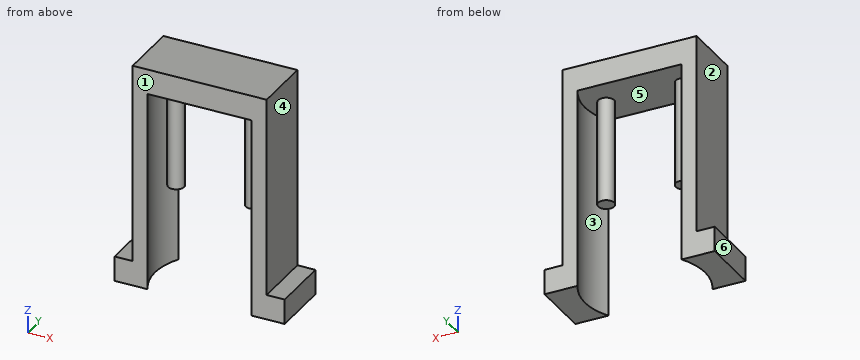
from build123d import *

# Parameters (mm, degrees)
BOSS_EXTRU_2_DEPTH = 5
BOSS_EXTRU_3_DEPTH = 35
ESQUISSE7_W        = 13.392304845
ESQUISSE7_H        = 12
ESQUISSE7_R        = 1.6
BOSS_EXTRU_4_DEPTH = 5
BOSS_EXTRU_5_START = -26
ESQUISSE9_R        = 1.6
BOSS_EXTRU_5_DEPTH = 26


with BuildPart() as part:
    # Esquisse5 → Boss.-Extru.2 (new body)
    with BuildSketch(Plane.XY):
        with BuildLine():
            Line((-17, 6), (-17, -6))
            Line((-17, -6), (-10.392304845, -6))
            ThreePointArc((-10.392304845, -6), (-12, 0), (-10.392304845, 6))
            Line((-10.392304845, 6), (-17, 6))
        make_face()
    boss_extru_2 = extrude(amount=BOSS_EXTRU_2_DEPTH)

    # Esquisse6 → Boss.-Extru.3 (add)
    with BuildSketch(Plane.XY.offset(5)):
        with BuildLine():
            Line((-13.392304845, 6), (-13.392304845, -6))
            Line((-13.392304845, -6), (-10.392304845, -6))
            ThreePointArc((-10.392304845, -6), (-12, 0), (-10.392304845, 6))
            Line((-10.392304845, 6), (-13.392304845, 6))
        make_face()
    boss_extru_3 = extrude(amount=BOSS_EXTRU_3_DEPTH)

    # Esquisse7 → Boss.-Extru.4 (add)
    with BuildSketch(Plane.XY.offset(40)):
        with Locations((-6.696152422, 0)):
            Rectangle(ESQUISSE7_W, ESQUISSE7_H)
        with Locations((-7.75, 0)):
            Circle(ESQUISSE7_R, mode=Mode.SUBTRACT)
    boss_extru_4 = extrude(amount=BOSS_EXTRU_4_DEPTH)

    # Symétrie9: Boss.-Extru.4 across plane
    add(boss_extru_4.mirror(Plane(origin=(0, 0, 0), x_dir=(0, 0, 1), z_dir=(1, 0, 0))))

    # Symétrie10: Boss.-Extru.3 across plane
    add(boss_extru_3.mirror(Plane(origin=(0, 0, 0), x_dir=(0, 0, 1), z_dir=(1, 0, 0))))

    # Symétrie11: Boss.-Extru.2 across plane
    add(boss_extru_2.mirror(Plane(origin=(0, 0, 0), x_dir=(0, 0, 1), z_dir=(1, 0, 0))))

    # Esquisse9 → Boss.-Extru.5 (add)
    with BuildSketch(Plane.XY.offset(45).offset(BOSS_EXTRU_5_START)):
        with Locations((-7.75, 0)):
            Circle(ESQUISSE9_R)
    boss_extru_5 = extrude(amount=BOSS_EXTRU_5_DEPTH)

    # Symétrie12: Boss.-Extru.5 across plane
    add(boss_extru_5.mirror(Plane(origin=(0, 0, 0), x_dir=(0, 0, 1), z_dir=(1, 0, 0))))


solid = part.part
Source: CAD feature listing. Evaluate the final solid. Frame: model axes, mm. Face numbers are marked on the shaded views. A direction names the side the tool comes from. Coordinates: 2 decimals unless noted, no trailing zeros. Order: outer loops, then holes, each group sorted by start corner. A loop starts at its lowest first (then second) coordinate and runs counter-clockwise, first axis right, second up. Notation, with made-up numbers: M 70.25,78.25 L 104.25,78.25 A12 cw 104.25,96.25 Z; hole C 30.25,-18 d5. An arc over 180 degrees is marked long. Write each question's results on one line, items separated by ' | '. Start each with the question number.
1. Section A-A, the plane z = 15. Return the cut outline in (x, y), then the cut area to 3 significant figures.
2. Section D-D, the plane x = -7.75. Return the cut outline in (y, z).
3. Reachability of the marked faces 4, 5 and 6 from +Z, -Z, +X, -X, +Y, -Y: full face, straight path, thin tool, end or side. Return the list, or none.
4. Section C-C, the plane y = 0. Return the cut outline in (x, z).
5. Draft query along X for the marked faces 1, 2 and 3. Return one class per face: +X half, -X half, draft (parallel to the pull), parting line (faces both ways), or undercut.
6. Pin query (flat end, axial travel): pin 1 (5 mm diameter, centred on y = 1.5, z = 22, fed in from -X); pin 2 (1 mm diameter, centred on x = 7.5, y = -0.5, fed in from -Z); pin 3 (10 mm diameter, centred on x = 5, z = 31.5, fed in from -Y). Return the tip coordinate at first contact, or that it passes through.
7. Material intervals for L1, parallel to X at y = -1, z = 19.5; L2, parallel to X at y = -1.25, z = 23; L3, parallel to X at y = -0.5, z = 6.5, sorted ascending.
8. Section B-B, the plane z = 38.5. Return the cut outline in (x, y).
Solution:
1) outline: M -13.39,-6 L -10.39,-6 A12 cw -10.39,6 L -13.39,6 Z; M 10.39,-6 L 13.39,-6 L 13.39,6 L 10.39,6 A12 cw Z | area: 45.9 mm²
2) outline: M -6,40 L -1.6,40 L -1.6,19 L 1.6,19 L 1.6,40 L 6,40 L 6,45 L -6,45 Z
3) face 4: +Z, +X, +Y, -Y | face 5: -Z | face 6: +Z, -Z, -X, +Y, -Y
4) outline: M -17,0 L -12,0 L -12,40 L -9.35,40 L -9.35,19 L -6.15,19 L -6.15,40 L 6.15,40 L 6.15,19 L 9.35,19 L 9.35,40 L 12,40 L 12,0 L 17,0 L 17,5 L 13.39,5 L 13.39,45 L -13.39,45 L -13.39,5 L -17,5 Z
5) face 1: draft | face 2: -X half | face 3: undercut
6) pin 1: x = -13.39 | pin 2: z = 19 | pin 3: y = -1.6
7) L1: -13.39 to -11.96, -9 to -6.5, 6.5 to 9, 11.96 to 13.39 | L2: -13.39 to -11.93, -8.75 to -6.75, 6.75 to 8.75, 11.93 to 13.39 | L3: -13.39 to -11.99, 11.99 to 13.39
8) outline: M -13.39,-6 L -10.39,-6 A12 cw -10.39,6 L -13.39,6 Z; C -7.75,0 d3.2; C 7.75,0 d3.2; M 10.39,-6 L 13.39,-6 L 13.39,6 L 10.39,6 A12 cw Z
